```python
from build123d import *

# Parameters (mm, degrees)
F1_DEPTH      = 6
F2_W          = 3.45
F2_H          = 0.85
F3_DEPTH      = 0.1
F3_DEPTH_BACK = 3.79
F4_R          = 0.3
F5_DEPTH      = 8


with BuildPart() as f1:
    # F0 (on Top) → F1 (new body)
    with BuildSketch(Plane.XY):
        Polygon((-98.6413434148, -69.7821304202), (-98.6413434148, -79.5412585139), (-87.0413434148, -79.5412585139), (-87.0413434148, -68.7412585139), (-91.0413434148, -68.7412585139), (-91.0413434148, -76.5412585139), (-94.6413434148, -76.5412585139), (-94.6413434148, -68.7412585139), (-97.1413434148, -68.7412585139), align=None)
    extrude(amount=F1_DEPTH)

    # F2 (on face) → F3 (cut, two sides)
    with BuildSketch(Plane.YZ.offset(-94.6413434148)) as f3_sk:
        with Locations((-70.4662585139, 3)):
            Rectangle(F2_W, F2_H)
    extrude(amount=-F3_DEPTH, mode=Mode.SUBTRACT)
    extrude(f3_sk.sketch, amount=F3_DEPTH_BACK, mode=Mode.SUBTRACT)

    # F4 (on face) → F5 (join)
    with BuildSketch(Plane.XZ.offset(79.5412585139)):
        with Locations((-96.2913434148, 4.15)):
            Circle(F4_R)
        with Locations((-96.2913434148, 1.85)):
            Circle(F4_R)
        with Locations((-89.3913434148, 4.15)):
            Circle(F4_R)
        with Locations((-89.3913434148, 1.85)):
            Circle(F4_R)
    extrude(amount=F5_DEPTH)


solid = f1.part
```
CAD build for the part. Positions are in the model's coordinates, mm. A direction names the side the tool comes from. Coordinates: 2 decimals unless noted, no trailing zeros. Order: outer loops, then holes, each group sorted by start corner. A loop starts at its lowest first (then second) coordinate and runs counter-clockwise, first axis right, second up.
(1) Which spindle directions (+Z, -Z, +X, -X, +Y, -Y) get a long thin tool onto all of the face, cutting with end or side? Do faces 5 (the face through (-90, -74, 6)), 6 (the face through (-91.041, -73, 3)). Say none if no direction does.
Solution:
face 5: +Z, +X, -X, +Y, -Y
face 6: +Z, -Z, +Y
(2) Saw through at B-B, the plane y = -85.75. Write the cut outline in (x, z), and give its area (3 significant figures).
Solution:
outline: circle Ø0.6 at (-96.29, 1.85); circle Ø0.6 at (-96.29, 4.15); circle Ø0.6 at (-89.39, 1.85); circle Ø0.6 at (-89.39, 4.15)
area: 1.13 mm2
(3) Pin check, flat tips, straight feed: pin 1 Ø1 at (x, y) = (-96.5, -84) entering from -Z; pin 2 Ø1.8 at (x, z) = (-94, 4) entering from -Y. Stop position of each tip, or through.
Solution:
pin 1: stops at z = 1.55
pin 2: stops at y = -79.54
(4) Saw through at D-D, the plane z = 5.25. Write the cut outline in (x, y).
Solution:
outline: (-98.64, -79.54) - (-87.04, -79.54) - (-87.04, -68.74) - (-91.04, -68.74) - (-91.04, -76.54) - (-94.64, -76.54) - (-94.64, -68.74) - (-97.14, -68.74) - (-98.64, -69.78) - close
(5) Mould opens along Z. For faces 1 (the face through (-90, -74, 0)), 2 (the face through (-97.881, -69.254, 2.958)), 3 (the face through (-94.741, -70, 3)), 4 (the face through (-90.851, -70, 3)) say: released by +Z, released by -Z, zero draft, split by the parting line, or undercut.
Solution:
face 1: released by -Z
face 2: zero draft
face 3: undercut
face 4: undercut
(6) Saw through at C-C, the plane x = -90. Write the cut outline in (y, z), and give its area (3 significant figures).
Solution:
outline: (-79.54, 0) - (-68.74, 0) - (-68.74, 6) - (-79.54, 6) - close
area: 64.8 mm2
(7) Saw through at A-A, the plane z = 1.85. Write the cut outline in (x, y).
Solution:
outline: (-98.64, -79.54) - (-96.59, -79.54) - (-96.59, -87.54) - (-95.99, -87.54) - (-95.99, -79.54) - (-89.69, -79.54) - (-89.69, -87.54) - (-89.09, -87.54) - (-89.09, -79.54) - (-87.04, -79.54) - (-87.04, -68.74) - (-91.04, -68.74) - (-91.04, -76.54) - (-94.64, -76.54) - (-94.64, -68.74) - (-97.14, -68.74) - (-98.64, -69.78) - close
(8) Drill centre lines: L1, parallel to X at y = -72.75, z = 2.2; L2, parallel to X at y = -82, z = 4.2; L3, parallel to Y at x = -95, z = 0.3. Where is each one in solid material? Low to high.
Solution:
L1: x = -98.64 to -94.64, -91.04 to -87.04
L2: x = -96.59 to -96, -89.69 to -89.1
L3: y = -79.54 to -68.74
